Can you work these out from the model? Positions are in its coordinate system, mm. A direction names the side the tool comes from. Round coordinates to 2 decimals unless told otherwise and drop trailing zeros. Write each loop counter-clockwise with the first axis right and the second up, starting at its lowest first coordinate (ties: lowest second). Pieces come first, ordered by that corner, then holes. Notation, with made-up numbers: M -32.5,10 L 6.5,10 A27 ccw 6.5,46 Z; hole C -14.5,70.5 d11. An arc over 180 degrees is marked long. Answer in a Markdown table with one row per item. Add a question column.
(1) I'm going to push flat-ended pins straight in: pin 1 (2 mm diameter, centred on y = 4, z = -6, fed in from +X); pin 2 (6 mm diameter, centred on x = -21.5, z = -5.5, fed in from +Y); pin 3 (5 mm diameter, centred on y = 24, z = -6, fed in from -X); pin 4 (3 mm diameter, centred on y = 6, z = -2, fed in from -X). Where does each tip first touch, or does it pass through?
(2) If we mould it in two halves opening along Y, with no side actions, what happens to faces 3 (the face through (-1.52, 29.4, -0.57)), 4 (the face through (-2.5, 8.7, 0)), 5 (the face through (-1.5, 12.1, -8)), 6 (the face through (-1.5, 22.8, -7.6))? For each: released by +Y, released by -Y, zero draft, split by the parting line, or undercut.
(3) Suppose I cut it at B-B, the plane y = 12. Write out the boundary of the cut face in (x, z), then the cut area to 3 significant figures.
(4) For faces 1 (the face through (-3, 17, -6)), 2 (the face through (-1.203, 1.141, -5.916)), which set-ups out of +Z, -Z, +X, -X, +Y, -Y let a thin tool reach every point of the face, with its end or its side?
(5) If I drill on probe 1 along X at (y, z) = (1.1, -6) (3 decimals); probe 2 along Y at (x, z) = (-19.25, -9.5); probe 3 along Z at (x, y) = (-0.65, 24), over which ranges is the centre line in solid material (lowest first)?
(6) Suppose I cut it at C-C, the plane x = -24. Write out the boundary of the cut face in (y, z), then the cut area to 3 significant figures.
(7) Suppose I cut it at A-A, the plane z = -6. Count the separate pieces of the cut face and the enclosed holes in it, then the cut area to 3 significant figures.
(8) Suppose I cut it at D-D, the plane x = -17.75. Write out the boundary of the cut face in (y, z).
Autodesk Inventor part; units mm, degrees
ref_plane "YZ Plane" through (0, 0, 0) normal (1, 0, 0) x (0, 1, 0)
ref_plane "XZ Plane" through (0, 0, 0) normal (0, 1, 0) x (-1, 0, 0)
ref_plane "XY Plane" through (0, 0, 0) normal (0, 0, 1) x (1, 0, 0)
sketch "Sketch1" plane through (0, 0, 0) normal (0, 1, 0) x (-1, 0, 0)
  line L0 (0, 0) -> (30, 0)
  line L1 (30, 0) -> (30, -12)
  line L2 (30, -12) -> (0, -12)
  line L3 (0, -12) -> (0, 0)
  dimension "d0" = 30
  dimension "d1" = 12
extrude "Extrusion1" add sketch "Sketch1" along normal blind 3
sketch "Sketch2" plane through (0, 3, 0) normal (0, 1, 0) x (1, 0, 0)
  line L0 (0, 0) -> (0, 12)
  line L1 (0, 12) -> (-30, 12)
  line L2 (0, 0) -> (-3, 0)
  line L3 (-3, 0) -> (-3, 12)
  line L4 (-3, 12) -> (0, 12)
  line L5 (0, 12) -> (0, 0)
  dimension "d4" = 3
extrude "Extrusion2" add sketch "Sketch2" along normal blind 27
sketch "Sketch4" plane through (0, 3, 0) normal (0, 1, 0) x (1, 0, 0)
  line L0 (-45.2087, 6) -> (21.2087, 6) construction
  line L1 (-30, 12) -> (-30, 0)
  line L2 (0, 0) -> (0, 12)
  point P0 (-30, 6)
  point P1 (-24, 6)
  point P2 (-12, 6)
  dimension "d7" = 12
  dimension "d9" = 18
hole "Hole1" at (-24, 3, -6) at (-12, 3, -6) direction (0, -1, 0) diameter 3.7 end through all countersink diameter 7 countersink angle 90
sketch "Sketch5" plane through (-3, 3, -12) normal (-1, 0, 0) x (0, 0, 1)
  line L0 (6, -9.8393) -> (6, 36.305) construction
  line L1 (0, -3) -> (12, -3)
  line L2 (0, 27) -> (12, 27)
  point P0 (6, -3)
  point P1 (6, 9)
  point P2 (6, 21)
  dimension "d17" = 12
  dimension "d18" = 18
hole "Hole2" at (-3, 12, -6) at (-3, 24, -6) direction (1, 0, 0) diameter 3.7 end through all countersink diameter 7 countersink angle 90
fillet "Fillet1" radius 2 5 edges at (-1.5, 30, -12) (-1.5, 30, 0) (-3, 3, -6) (-30, 1.5, 0) (-30, 1.5, -12)
fillet "Fillet2" radius 4 1 edges at (0, 0, -6)
properties part number "Right Bracket 30mm RS749-1686"
Calculated:
| question | item | result |
|---|---|---|
| 1 | pin 1 | x = 0 |
| 1 | pin 2 | y = 3 |
| 1 | pin 3 | x = -2 |
| 1 | pin 4 | x = -3.06 |
| 2 | face 3 | released by +Y |
| 2 | face 4 | zero draft |
| 2 | face 5 | undercut |
| 2 | face 6 | undercut |
| 3 | outline | M -3,-12 L 0,-12 L 0,-7.85 L -1.35,-7.85 L -3,-9.5 Z; M -3,-2.5 L -1.35,-4.15 L 0,-4.15 L 0,0 L -3,0 Z |
| 3 | area | 22.2 mm² |
| 4 | face 1 | +Z, -Z, -X, +Y |
| 4 | face 2 | +Z, -Z, +X, -Y |
| 5 | probe 1 | -30 to -25.85, -22.15 to -13.85, -10.15 to -1.245 |
| 5 | probe 2 | 0 to 3 |
| 5 | probe 3 | -12 to -7.85, -4.15 to 0 |
| 6 | outline | M 0,-12 L 3,-12 L 3,-9.5 L 1.35,-7.85 L 0,-7.85 Z; M 0,-4.15 L 1.35,-4.15 L 3,-2.5 L 3,0 L 0,0 Z |
| 6 | area | 22.2 mm² |
| 7 | separate pieces | 5 |
| 7 | enclosed holes | 0 |
| 7 | area | 113 mm² |
| 8 | outline | M 0,-12 L 3,-12 L 3,0 L 0,0 Z |
